Part model, mm, in its own coordinate system. Face numbers are marked on the shaded views. A direction names the side the tool comes from. Round coordinates to 2 decimals unless told otherwise and drop trailing zeros. Write each loop counter-clockwise with the first axis right and the second up, starting at its lowest first coordinate (ties: lowest second). Pieces come first, ordered by that corner, then holes.
```python
from build123d import *

# Parameters (mm, degrees)
BOSS_EXTRUDE1_DEPTH = 165.1
SKETCH2_R           = 12.7
CUT_EXTRUDE1_DEPTH  = 11.938


with BuildPart() as part:
    # Sketch1 → Boss-Extrude1 (new body)
    with BuildSketch(Plane(origin=(0, 0, 0), x_dir=(0, 0, -1), z_dir=(1, 0, 0))):
        with BuildLine():
            Line((-21.9075, -6.6675), (-21.9075, 9.2075))
            Line((-21.9075, 9.2075), (-21.9075, 12.7))
            Line((-21.9075, 12.7), (-25.4, 12.7))
            Line((-25.4, 12.7), (-25.4, -12.7))
            Line((-25.4, -12.7), (25.4, -12.7))
            Line((25.4, -12.7), (25.4, 12.7))
            Line((25.4, 12.7), (21.9075, 12.7))
            Line((21.9075, 12.7), (21.9075, 9.2075))
            Line((21.9075, 9.2075), (21.9075, -6.6675))
            ThreePointArc((21.9075, -6.6675), (21.163551224, -8.463551224), (19.3675, -9.2075))
            Line((19.3675, -9.2075), (-19.3675, -9.2075))
            ThreePointArc((-19.3675, -9.2075), (-21.163551224, -8.463551224), (-21.9075, -6.6675))
        make_face()
    extrude(amount=-BOSS_EXTRUDE1_DEPTH)

    # Sketch2 → Cut-Extrude1 (cut)
    with BuildSketch(Plane.XZ.offset(12.7)):
        with Locations(Location((-82.55, 0, 0), (0, 0, 270))):
            Circle(SKETCH2_R)
    extrude(amount=-CUT_EXTRUDE1_DEPTH, mode=Mode.SUBTRACT)


solid = part.part
```
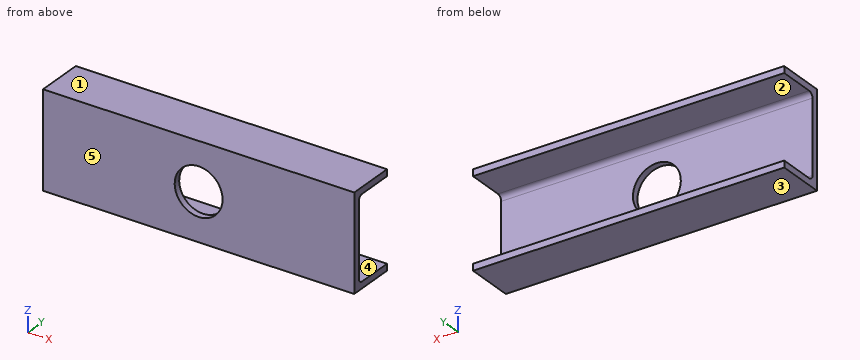
Q1. Cut at A-A on x = -82.55. Write the cut outline in (y, z), plus the area to 3 significant figures.
Values follow:
outline: (-12.7, -25.4) - (12.7, -25.4) - (12.7, -21.91) - (-6.67, -21.91) arc R2.54 cw to (-9.21, -19.37) - (-9.21, -12.7) - (-12.7, -12.7) - close; (-12.7, 12.7) - (-9.21, 12.7) - (-9.21, 19.37) arc R2.54 cw to (-6.67, 21.91) - (12.7, 21.91) - (12.7, 25.4) - (-12.7, 25.4) - close
area: 245 mm2
Q2. Cut at C-C on y = 8.5. Write the cut outline in (x, z), plus the area to 3 significant figures.
Values follow:
outline: (-165.1, -25.4) - (0, -25.4) - (0, -21.91) - (-165.1, -21.91) - close; (-165.1, 21.91) - (0, 21.91) - (0, 25.4) - (-165.1, 25.4) - close
area: 1,150 mm2
Q3. Drop a flat-ended pin along its axis: pin 1 (12 mm diameter, centred on x = -53.5, z = -10.5, fed in from +Y). Give the stop position or say it passes through.
Values follow:
pin 1: stops at y = -9.21
Q4. Wall check: L1, parallel to Z at x = -93, y = 2; L2, parallel to X at y = -11.7, z = 0; L3, parallel to Y at x = -13.5, z = -13. Give the ranges that are in metal, low to high.
Values follow:
L1: z = -25.4 to -21.91, 21.91 to 25.4
L2: x = -165.1 to -95.25, -69.85 to 0
L3: y = -12.7 to -9.21
Q5. Cut at D-D on x = -142.5. Write the cut outline in (y, z), plus the area to 3 significant figures.
Values follow:
outline: (-12.7, -25.4) - (12.7, -25.4) - (12.7, -21.91) - (-6.67, -21.91) arc R2.54 cw to (-9.21, -19.37) - (-9.21, 19.37) arc R2.54 cw to (-6.67, 21.91) - (12.7, 21.91) - (12.7, 25.4) - (-12.7, 25.4) - close
area: 333 mm2
Q6. Cut at B-B on z = 0. Write the cut outline in (x, y), plus the area to 3 significant figures.
Values follow:
outline: (-165.1, -12.7) - (-95.25, -12.7) - (-95.25, -9.21) - (-165.1, -9.21) - close; (-69.85, -12.7) - (0, -12.7) - (0, -9.21) - (-69.85, -9.21) - close
area: 488 mm2
Q7. Which spindle directions (+Z, -Z, +X, -X, +Y, -Y) get a long thin tool onto all of the face, cutting with end or side? Do the marked faces 4 and 5. Say none if no direction does.
Values follow:
face 4: +X, -X, +Y
face 5: +Z, -Z, +X, -X, -Y
Q8. Mould opens along Z. For the marked faces 1, 2 and 3 say: +Z half, -Z half, draft (parallel to the pull), parting line (faces both ways), or undercut.
Values follow:
face 1: +Z half
face 2: undercut
face 3: -Z half
